Check sheet for the drawn part. Datum: minimum x, y, z corner. Units: mm. Give positions to 0.01 mm unless a question says otherwise; leave off trailing zeros. Order: outer loops, then holes, each group sorted by start corner. A loop starts at its lowest first (then second) coordinate and runs counter-clockwise, first axis right, second up. Notation, with made-up numbers: M 89,66 L 101,66 A15 ccw 101,78 Z; hole C 29,55 d6. An arc over 180 degrees is marked long. Answer as CSV lines item,"result". Start each with the question number.
Q1. Section check B-B, the plane x = 2.2. Count the separate pieces of the cut face and the enclosed holes in it, then the cut area to 3 significant figures.
Q2. Section check C-C, the plane y = 94. Record the boundary of the cut face in (x, z) (1 decimal).
Q3. Section check A-A, the plane z = 47.5. Record the boundary of the cut face in (x, y) (1 decimal).
Q4. Thickness scan on line 1 (Y direction, x = 0.5, z = 43.5); line 2 (Z direction, x = 2.3, y = 87) (1 decimal); line 3 (Z direction, x = 2.05, y = 50.5) (1 decimal). Record the ranges inside material, lowest first.
Q5. Go/stop test with flat-tipped pins: pin 1 (1.4 mm diameter, centred on x = 2, y = 158, fed in from +Z); pin 2 (5 mm diameter, centred on y = 29, z = 21.5, fed in from -X); pin 3 (2 mm diameter, centred on x = 3.5, z = 17.5, fed in from +Y). Record where each tip stops, or that it passes through.
Q6. Section check D-D, the plane z = 69. Record the boundary of the cut face in (x, y) (1 decimal).
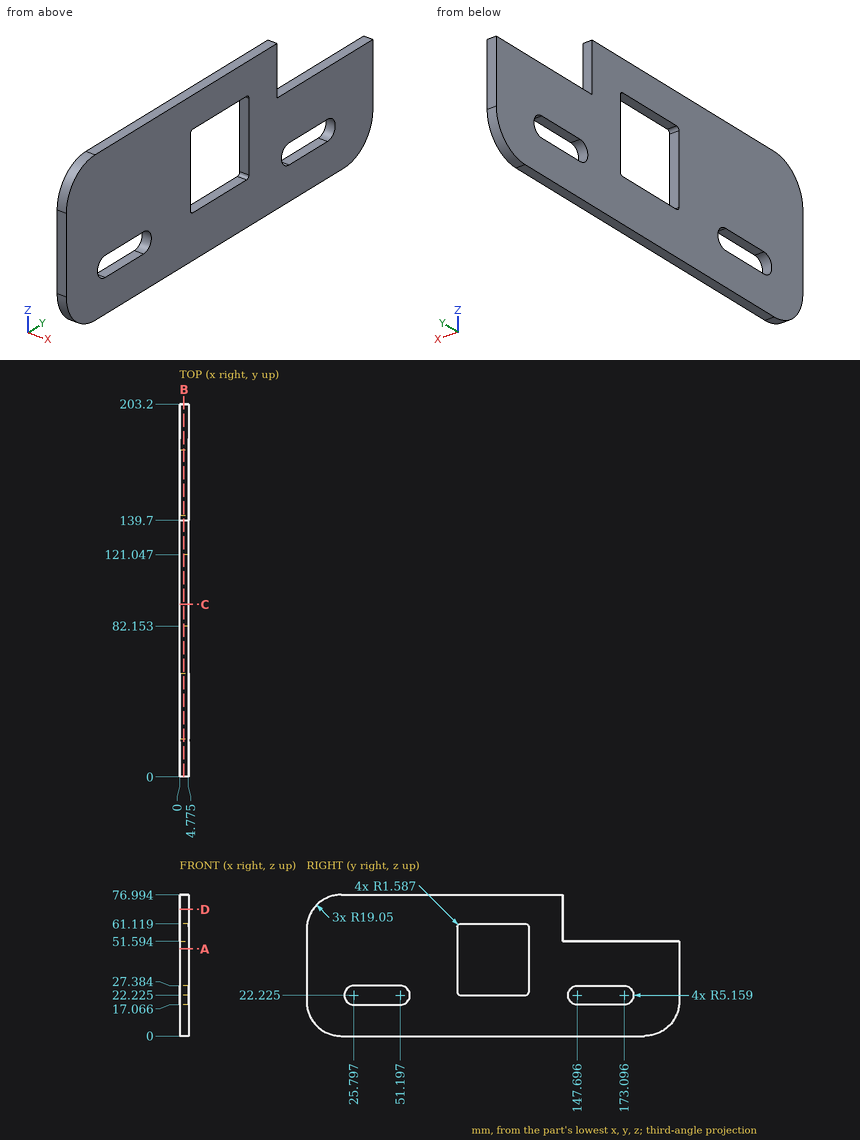
Answer block:
1,separate pieces,"1"
1,enclosed holes,"3"
1,area,"11,600 mm2"
2,outline,"M 0,0 L 4.8,0 L 4.8,22.2 L 0,22.2 Z; M 0,61.1 L 4.8,61.1 L 4.8,77 L 0,77 Z"
3,outline,"M 0,0 L 4.8,0 L 4.8,82.2 L 0,82.2 Z; M 0,121 L 4.8,121 L 4.8,203.2 L 0,203.2 Z"
4,line 1,"y = 0 to 82.15, 121.05 to 203.2"
4,line 2,"z = 0 to 22.2, 61.1 to 77"
4,line 3,"z = 0 to 17.1, 27.4 to 77"
5,pin 1,"stops at z = 51.59"
5,pin 2,"passes through"
5,pin 3,"stops at y = 203.19"
6,outline,"M 0,3.5 L 4.8,3.5 L 4.8,139.7 L 0,139.7 Z"
